Geometry check sheet. Reference: the model listing, model coordinates, mm. Face numbers are marked on the shaded views. A direction names the side the tool comes from. Give positions to 0.01 mm unless a question says otherwise; leave off trailing zeros. Order: outer loops, then holes, each group sorted by start corner. A loop starts at its lowest first (then second) coordinate and runs counter-clockwise, first axis right, second up. Notation, with made-up numbers: M 76.5,-13 L 90.5,-13 A28 ccw 90.5,24 Z; hole C 8,26.5 d7. An arc over 180 degrees is marked long. Answer as CSV lines item,"result". Start each with the question number.
```python
from build123d import *

# Parameters (mm, degrees)
SKETCH1_R                     = 3.048
SKETCH1_R_2                   = 1.651
BOSS_EXTRUDE1_DEPTH           = 10.16
CIRPATTERN1_COUNT             = 2
CIRPATTERN1_ANGLE             = 25
CIRPATTERN2_COUNT             = 3
CIRPATTERN2_COPY_1_SKETCH_R   = 3.048
CIRPATTERN2_COPY_1_SKETCH_R_2 = 1.651
CIRPATTERN2_COPY_1_DEPTH      = 10.16
CIRPATTERN2_COPY_2_SKETCH_R   = 3.048
CIRPATTERN2_COPY_2_SKETCH_R_2 = 1.651
CIRPATTERN2_COPY_2_DEPTH      = 10.16
FILLET1_R                     = 15.24
CUT_EXTRUDE1_DEPTH            = 9.398
BOSS_EXTRUDE3_REACH           = 49.452
SKETCH7_W                     = 10.16
SKETCH7_H                     = 19.663186572
CUT_EXTRUDE3_START            = -1.198457
SKETCH8_W                     = 10.16
SKETCH8_H                     = 19.663186572
CUT_EXTRUDE3_DEPTH            = 1.198457
CUT_EXTRUDE2_REACH            = 49.452
CUT_EXTRUDE2_END_RADIUS       = 3.048
SKETCH5_R                     = 2.159


with BuildPart() as part:
    # Sketch1 → Boss-Extrude1 (new body)
    with BuildSketch(Plane.XY):
        with BuildLine():
            Line((-17.78, 5.08), (0, 5.08))
            ThreePointArc((0, 5.08), (5.08, 0), (0, -5.08))
            Line((0, -5.08), (-17.78, -5.08))
            ThreePointArc((-17.78, -5.08), (-22.86, 0), (-17.78, 5.08))
        make_face()
        Circle(SKETCH1_R, mode=Mode.SUBTRACT)
        with Locations((-17.78, 0)):
            Circle(SKETCH1_R_2, mode=Mode.SUBTRACT)
    boss_extrude1 = extrude(amount=BOSS_EXTRUDE1_DEPTH)

    # CirPattern1: Boss-Extrude1 ×2 about axis
    cirpattern1_axis = Axis((0, 0, 10.16), (0, 0, 1))
    for i in range(1, CIRPATTERN1_COUNT):
        add(boss_extrude1.rotate(cirpattern1_axis, i * CIRPATTERN1_ANGLE / (CIRPATTERN1_COUNT - 1)))

    # CirPattern2: Boss-Extrude1 ×3 about axis
    cirpattern2_axis = Axis((0, 0, 0), (0, 0, 1))
    for i in range(1, CIRPATTERN2_COUNT):
        add(boss_extrude1.rotate(cirpattern2_axis, i * 360 / CIRPATTERN2_COUNT))

    # CirPattern2 copy 1 sketch → CirPattern2 copy 1 (add)
    with BuildSketch(Plane(origin=(0, 0, 0), x_dir=(-0.8191520442889921, 0.5735764363510454, 0), z_dir=(0, 0, 1))):
        with BuildLine():
            Line((-17.78, 5.08), (0, 5.08))
            ThreePointArc((0, 5.08), (5.08, 0), (0, -5.08))
            Line((0, -5.08), (-17.78, -5.08))
            ThreePointArc((-17.78, -5.08), (-22.86, 0), (-17.78, 5.08))
        make_face()
        Circle(CIRPATTERN2_COPY_1_SKETCH_R, mode=Mode.SUBTRACT)
        with Locations((-17.78, 0)):
            Circle(CIRPATTERN2_COPY_1_SKETCH_R_2, mode=Mode.SUBTRACT)
    extrude(amount=CIRPATTERN2_COPY_1_DEPTH)

    # CirPattern2 copy 2 sketch → CirPattern2 copy 2 (add)
    with BuildSketch(Plane(origin=(0, 0, 0), x_dir=(-0.0871557427476577, -0.9961946980917455, 0), z_dir=(0, 0, 1))):
        with BuildLine():
            Line((-17.78, 5.08), (0, 5.08))
            ThreePointArc((0, 5.08), (5.08, 0), (0, -5.08))
            Line((0, -5.08), (-17.78, -5.08))
            ThreePointArc((-17.78, -5.08), (-22.86, 0), (-17.78, 5.08))
        make_face()
        Circle(CIRPATTERN2_COPY_2_SKETCH_R, mode=Mode.SUBTRACT)
        with Locations((-17.78, 0)):
            Circle(CIRPATTERN2_COPY_2_SKETCH_R_2, mode=Mode.SUBTRACT)
    extrude(amount=CIRPATTERN2_COPY_2_DEPTH)

    # Fillet1
    # the kernel refuses this fillet: 15.24 mm, written as the material it adds along each edge
    with BuildSketch(Plane(origin=(-4.654962364, 5.08, 0), x_dir=(0.0874683738412008, 0.9961672969825781, 0), z_dir=(0, 0, 1)), Plane(origin=(6.726890233, 1.491315661, 0), x_dir=(0.81897199868559, -0.5738334822654828, 0), z_dir=(0, 0, 1))) as fillet1_piece_1:
        with BuildLine():
            CenterArc((13.944774221, 15.227642174), FILLET1_R, 187.343482599, 80.348997025)
            Line((-1.17022312, 13.279705988), (-2.681722854, 13.084912369))
            ThreePointArc((-2.681722854, 13.084912369), (-2.666184659, 12.941431463), (-1.518158961, -0.133301802))
            Line((-1.518158961, -0.133301802), (0.000478276, -1.523999925))
            ThreePointArc((0.000478276, -1.523999925), (13.125515266, -1.5198809), (13.269806265, -1.522764217))
            Line((13.269806265, -1.522764217), (13.331166988, 0))
        make_face()
    extrude(amount=10.16)
    with BuildSketch(Plane(origin=(-2.071927869, -6.571315661, 10.16), x_dir=(-0.9064403725267903, -0.4223338147170952, 0), z_dir=(0, 0, -1))) as fillet1_piece_2:
        with BuildLine():
            CenterArc((13.944774221, -15.227642174), FILLET1_R, 92.307520375, 80.348997025)
            Line((-1.17022312, -13.279705988), (-2.681722854, -13.084912369))
            ThreePointArc((-2.681722854, -13.084912369), (-2.666184659, -12.941431463), (-1.518158961, 0.133301802))
            Line((-1.518158961, 0.133301802), (0.000478276, 1.523999925))
            ThreePointArc((0.000478276, 1.523999925), (13.125515266, 1.5198809), (13.269806265, 1.522764217))
            Line((13.269806265, 1.522764217), (13.331166988, 0))
        make_face()
    extrude(amount=10.16)

    # Sketch4 → Cut-Extrude1 (cut)
    with BuildSketch(Plane.XY.offset(10.16)):
        Polygon((4.024997463, 5.315159398), (5.894169969, -3.11613292), (9.117899385, -2.401449315), (7.248726879, 6.029843003), align=None)
    extrude(amount=-CUT_EXTRUDE1_DEPTH, mode=Mode.SUBTRACT)

    # Sketch7 → Boss-Extrude3 (add, up to next)
    with BuildSketch(Plane(origin=(16.68684539, 3.699384559, 0), x_dir=(0, 0, -1), z_dir=(0.9762960071199317, 0.21643961393811023, 0)), mode=Mode.PRIVATE) as boss_extrude3_sk1:
        with Locations((-5.08, 0)):
            Rectangle(SKETCH7_W, SKETCH7_H)
    boss_extrude3_tool1 = extrude(boss_extrude3_sk1.sketch, amount=-BOSS_EXTRUDE3_REACH, mode=Mode.PRIVATE) - part.part
    add(boss_extrude3_tool1.solids().sort_by_distance((16.686845, 3.699385, 5.08))[0])

    # Sketch8 → Cut-Extrude3 (cut)
    with BuildSketch(Plane(origin=(16.68684539, 3.699384559, 0), x_dir=(0, 0, -1), z_dir=(0.9762960071199318, 0.2164396139381102, 0)).offset(CUT_EXTRUDE3_START)):
        with Locations((-5.08, 0)):
            Rectangle(SKETCH8_W, SKETCH8_H)
    extrude(amount=CUT_EXTRUDE3_DEPTH, mode=Mode.SUBTRACT)

    # Cut-Extrude2: up to this cylinder (the profile starts outside it)
    cut_extrude2_end = Plane(origin=(0, 0, 5.08), z_dir=(0, 0, -1)) * Cylinder(CUT_EXTRUDE2_END_RADIUS, 106, mode=Mode.PRIVATE)
    # Sketch5 → Cut-Extrude2 (cut, up to the surface)
    with BuildSketch(Plane(origin=(16.68684539, 3.699384559, 0), x_dir=(0, 0, -1), z_dir=(0.9762960071199317, 0.21643961393811023, 0)), mode=Mode.PRIVATE) as cut_extrude2_sk1:
        with Locations(Location((-5.08, 0, 0), (0, 0, 90))):
            Circle(SKETCH5_R)
    cut_extrude2_tool1 = extrude(cut_extrude2_sk1.sketch, amount=-CUT_EXTRUDE2_REACH, mode=Mode.PRIVATE) - cut_extrude2_end
    add(cut_extrude2_tool1.solids().sort_by_distance((16.686845, 3.699385, 5.08))[0], mode=Mode.SUBTRACT)


solid = part.part
```
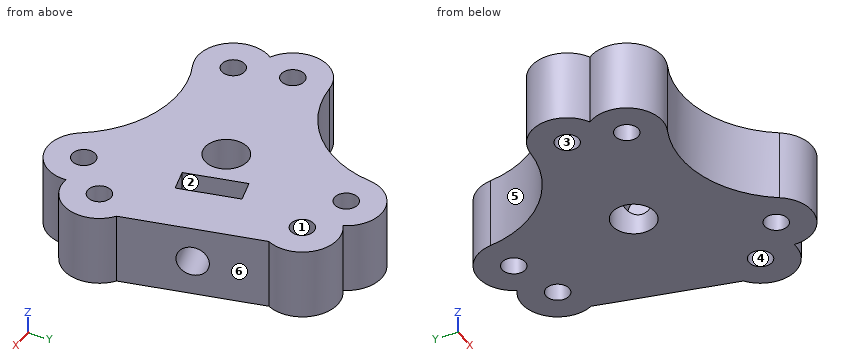
Item 1: Section check B-B on z = 8.25. Give the number of separate pieces and of enclosed holes in the cut face, then the cut area to 3 significant figures.
Item 2: Depth check by flat-ended pin: pin 1 Ø1.5 at (x, y) = (6, 2.5) entering from +Z; pin 2 Ø6 at (x, z) = (-10, 3) entering from +Y; pin 3 Ø6 at (y, z) = (-8, 5.5) entering from -X. Enter the tip coordinate at first touch or a pass-through.
Item 3: Scan lines: line 1 along X through (y, z) = (16.5, 5); line 2 along Y through (x, z) = (2, 6); line 3 along X through (y, z) = (4.5, 7.5). Record each from-to range of solid material in increasing order.
Item 4: Section check A-A on x = -15.5. Record the boundary of the cut face in (y, z).
Item 5: Section check D-D on z = 6. Record the boundary of the cut face in (x, y) (1 decimal), then the cut area to 3 significant figures.
Item 6: Draft check along X on the marked faces 3, 4, 5 and 6. Enter one of: pulls with the +X half, pulls with the -X half, needs draft (parallel to the pull), parting line crosses it, or undercut.
Item 7: Access from +Z, -Z, +X, -X, +Y, -Y to the whole of each face (thin tool, end or side, straight path). Record for the marked faces 1 and 2.
Numbers:
1,separate pieces,"1"
1,enclosed holes,"8"
1,area,"974 mm2"
2,pin 1,"z = 0.76"
2,pin 2,"y = 10.42"
2,pin 3,"x = -21.19"
3,line 1,"-3.85 to 0.43, 2.67 to 7.66, 10.12 to 13.85"
3,line 2,"-15.01 to -2.3, 2.44 to 16.12, 19.3 to 22.77"
3,line 3,"-20.14 to 4.21, 7.59 to 15.28"
4,outline,"M -12.56,0 L -9.05,0 L -9.05,10.16 L -12.56,10.16 Z; M -5.98,0 L 5.38,0 L 5.38,10.16 L -5.98,10.16 Z"
5,outline,"M -20.2,-4.5 A5.1 ccw -14.2,-12.2 A15.2 cw 4.6,-18.1 A5.1 ccw 14,-15.2 A5.1 ccw 17.6,-6.2 L 15.9,1.5 L 8.6,-0.1 L 9.1,-2.4 L 5.9,-3.1 L 5.4,-0.8 L 2.7,-1.4 A3 cw long 1.9,2.4 L 4.5,3 L 4,5.3 L 7.2,6 L 7.8,3.7 L 15.1,5.3 L 13.4,13 A5.1 ccw 6.2,19.7 A5.1 ccw -3.5,18.4 A15.2 cw -18,5.1 A5.1 ccw Z; hole C -17.8,0 d3.3; hole C -16.1,-7.5 d3.3; hole C 1.5,17.7 d3.3; hole C 8.9,-15.4 d3.3; hole C 8.9,15.4 d3.3; hole C 14.6,-10.2 d3.3"
5,area,"936 mm2"
6,face 3,"undercut"
6,face 4,"undercut"
6,face 5,"pulls with the -X half"
6,face 6,"pulls with the +X half"
7,face 1,"+Z, -Z"
7,face 2,"+Z"
